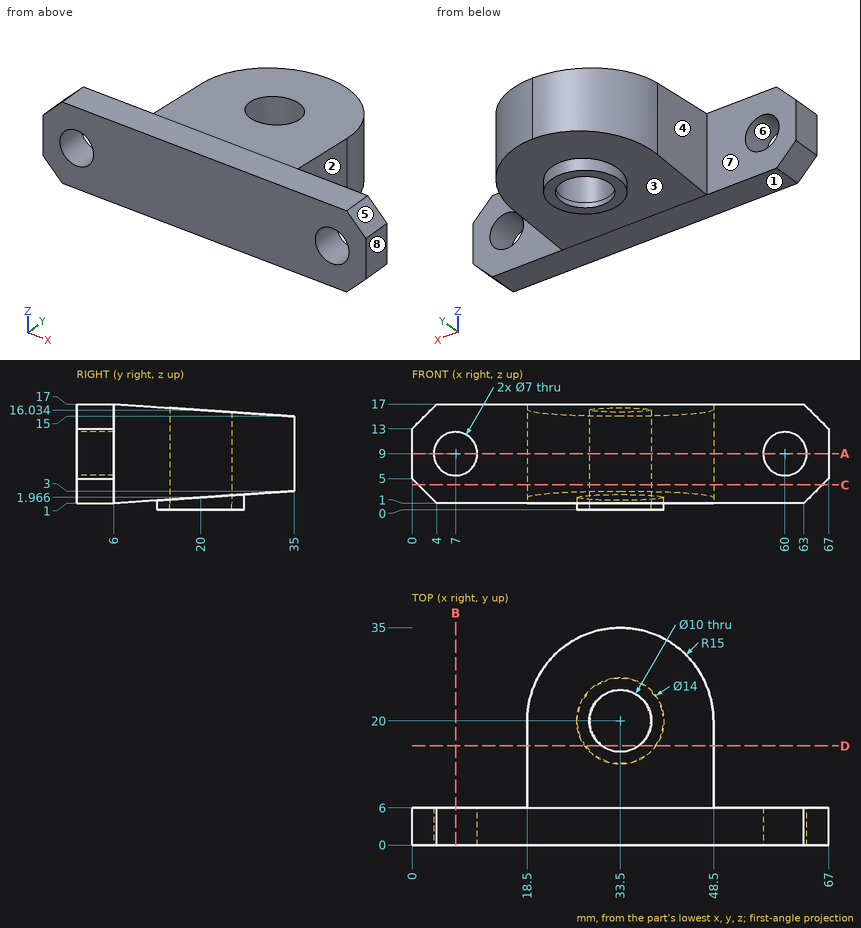
Study the drawing (mm; zero at the part's minimum x, y, z) and answer. A direction names the side the tool comes from. Coordinates: 2 decimals unless noted, no trailing zeros. Order: outer loops, then holes, each group sorted by start corner. A loop starts at its lowest first (then second) coordinate and runs counter-clockwise, first axis right, second up. Notation, with made-up numbers: (60.25, 87) -> (88.25, 87) arc R26 cw to (88.25, 101) -> close; hole circle Ø2 at (-28, -19.75). An arc over 180 degrees is marked (long way). Answer in a Markdown table with one row per item. Add a question column.
Item 1: Determine the mould class of the marked faces 6, 7 and 8 for opening direction X: +X half, -X half, draft (parallel to the pull), parting line (faces both ways), or undercut.
Item 2: Find section B-B (x = 7). Write down the section's boundary in (y, z).
Item 3: Find section D-D (y = 16). Write down the section's boundary in (x, z) (1 decimal), then the cut area to 3 significant figures.
Item 4: Find the intervals of material crossed by L1, parallel to X at y = 20, z = 10; L2, parallel to Z at x = 7, y = 4.55; L3, parallel to Y at x = 33.5, z = 12.75, in increasing order. Write a range as from..to.
Item 5: Find section A-A (z = 9). Write down the section's boundary in (x, y).
Item 6: Find section C-C (z = 4). Write down the section's boundary in (x, y).
Item 7: Which of the six approach directions +Z, -Z, +X, -X, +Y, -Y give full straight-line access (tool end or side, diameter ignored) to the marked faces 1, 2, 3, 4 and 5?
Item 8: Each of these flat-tipped pins is pushed along its axis until it touches: P1, Ø5, axis at x = 46.5, z = 10, coming from the +Y side; P2, Ø8, axis at x = 60, z = 9, coming from the +Y side; P3, Ø2, axis at x = 42.5, y = 23.5, coming from the +Z side; P4, Ø8, axis at x = 33.5, y = 20, coming from the -Z side. Where does it stop, or does it pass through?
Result set:
| question | item | result |
|---|---|---|
| 1 | face 6 | undercut |
| 1 | face 7 | draft |
| 1 | face 8 | +X half |
| 2 | outline | (0, 1) -> (6, 1) -> (6, 5.5) -> (0, 5.5) -> close; (0, 12.5) -> (6, 12.5) -> (6, 17) -> (0, 17) -> close |
| 3 | outline | (18.5, 1.7) -> (27.8, 1.7) -> (27.8, 0) -> (30.5, 0) -> (30.5, 16.3) -> (18.5, 16.3) -> close; (36.5, 0) -> (39.2, 0) -> (39.2, 1.7) -> (48.5, 1.7) -> (48.5, 16.3) -> (36.5, 16.3) -> close |
| 3 | area | 360 mm² |
| 4 | L1 | x = 18.5..28.5, 38.5..48.5 |
| 4 | L2 | z = 1..5.5, 12.5..17 |
| 4 | L3 | y = 0..15, 25..35 |
| 5 | outline | (0, 0) -> (3.5, 0) -> (3.5, 6) -> (0, 6) -> close; (10.5, 0) -> (56.5, 0) -> (56.5, 6) -> (48.5, 6) -> (48.5, 20) arc R15 ccw to (18.5, 20) -> (18.5, 6) -> (10.5, 6) -> close; (63.5, 0) -> (67, 0) -> (67, 6) -> (63.5, 6) -> close; hole circle Ø10 at (33.5, 20) |
| 6 | outline | (1, 0) -> (66, 0) -> (66, 6) -> (48.5, 6) -> (48.5, 20) arc R15 ccw to (18.5, 20) -> (18.5, 6) -> (1, 6) -> close; hole circle Ø10 at (33.5, 20) |
| 7 | face 1 | -Z, +X, -X, -Y |
| 7 | face 2 | +Z, -Z, +X, +Y |
| 7 | face 3 | -Z |
| 7 | face 4 | +Z, -Z, -X, +Y |
| 7 | face 5 | +Z, +X, +Y, -Y |
| 8 | P1 | stops at y = 30.71 |
| 8 | P2 | stops at y = 6 |
| 8 | P3 | stops at z = 15.86 |
| 8 | P4 | passes through |
